For this review, use the dimensioned drawing (mm, ordinates from the lowest corner) and the shaded views. A direction names the side the tool comes from. Coordinates: 2 decimals unless noted, no trailing zeros. Write each loop counter-clockwise with the first axis right and the second up, starting at its lowest first coordinate (ties: lowest second). Pieces come first, ordered by that corner, then holes. Notation, with made-up numbers: M 46,81 L 52,81 A13 ccw 52,104 Z; hole C 16.5,14 d2. An arc over 180 degrees is marked long. One line per question, with ' | ' between items.
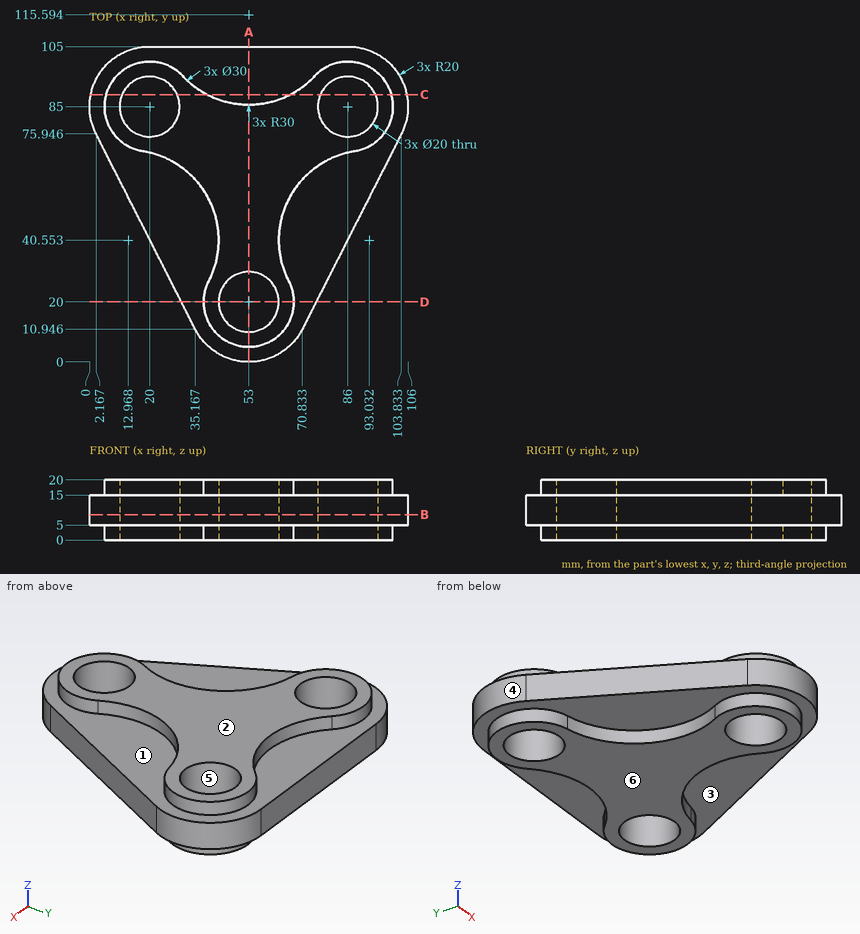
1. Take a section at A-A (x = 53). Write out the cut boundary in (y, z).
Answer sheet:
outline: M 0,5 L 5,5 L 5,0 L 10,0 L 10,20 L 5,20 L 5,15 L 0,15 Z; M 30,0 L 85.59,0 L 85.59,5 L 105,5 L 105,15 L 85.59,15 L 85.59,20 L 30,20 Z
2. Insertion check: pin 1 Ø12 at (x, z) = (91.5, 15.5) entering from -Y (1 decimal); pin 2 Ø16 at (x, y) = (53, 20) entering from +Z; pin 3 Ø12 at (y, z) = (73.5, 15) entering from -X; pin 4 Ø4 at (x, y) = (73.5, 26) entering from -Z. Each pin has a flat end and moves straight along its axis. Give the tip position at first contact, or say it passes through.
Answer sheet:
pin 1: y = 39.9 | pin 2: through | pin 3: x = 0.77 | pin 4: z = 5
3. Take a section at C-C (y = 89). Write out the cut boundary in (x, z) (1 decimal).
Answer sheet:
outline: M 0.4,5 L 5.5,5 L 5.5,0 L 10.8,0 L 10.8,20 L 5.5,20 L 5.5,15 L 0.4,15 Z; M 29.2,0 L 39.1,0 L 39.1,5 L 66.9,5 L 66.9,0 L 76.8,0 L 76.8,20 L 66.9,20 L 66.9,15 L 39.1,15 L 39.1,20 L 29.2,20 Z; M 95.2,0 L 100.5,0 L 100.5,5 L 105.6,5 L 105.6,15 L 100.5,15 L 100.5,20 L 95.2,20 Z
4. Tool access review of the marked faces 1, 2 and 3: name each direction out of +Z, -Z, +X, -X, +Y, -Y from which nothing blocks a thin tool from reaching the whole face with its end or side.
Answer sheet:
face 1: +Z | face 2: +Z, +X, -X, +Y, -Y | face 3: -Z
5. Draft analysis for pull direction X (two halves, no side actions). For the marked faces 4, 5 and 6, state which applies: pulls with the +X half, pulls with the -X half, needs draft (parallel to the pull), parting line crosses it, or undercut.
Answer sheet:
face 4: pulls with the -X half | face 5: undercut | face 6: needs draft
6. To check wall thickness, follow line 1 along Z through (x, y) = (81.5, 100.5); line 2 along X through (y, z) = (76.5, 11.25) (1 decimal); line 3 along X through (y, z) = (40.5, 18.5). State the ranges of each line that lie inside material, in increasing order. Write a range as [from, to].
Answer sheet:
line 1: [5, 15] | line 2: [1.9, 14.7], [25.3, 80.7], [91.3, 104.1] | line 3: [42.97, 63.03]
7. Take a section at B-B (z = 8.5). Write out the cut boundary in (x, y).
Answer sheet:
outline: M 2.17,75.95 L 35.17,10.95 A20 ccw 70.83,10.95 L 103.83,75.95 A20 ccw 86,105 L 20,105 A20 ccw Z; hole C 20,85 d20; hole C 53,20 d20; hole C 86,85 d20
8. Take a section at D-D (y = 20). Write out the cut boundary in (x, z), then the cut area to 3 significant figures.
Answer sheet:
outline: M 30.57,5 L 38,5 L 38,0 L 43,0 L 43,20 L 38,20 L 38,15 L 30.57,15 Z; M 63,0 L 68,0 L 68,5 L 75.43,5 L 75.43,15 L 68,15 L 68,20 L 63,20 Z | area: 349 mm^2
